Autodesk Inventor part; units mm, degrees
ref_plane "YZ Plane" through (0, 0, 0) normal (1, 0, 0) x (0, 1, 0)
ref_plane "XZ Plane" through (0, 0, 0) normal (0, 1, 0) x (-1, 0, 0)
ref_plane "XY Plane" through (0, 0, 0) normal (0, 0, 1) x (1, 0, 0)
sketch "Sketch1" plane through (0, 0, 0) normal (0, 0, 1) x (1, 0, 0)
  line L0 (-179.705, 0) -> (89.2175, 0)
  line L1 (0, -106.7147) -> (0, 106.7147)
  circle A0 centre (0, 0) radius 50.8 construction
  arc A1 (-12.7, 50.8248) -> (-12.7, -50.8248) centre (0, 0) ccw
  line L2 (0, -55.5625) -> (0, -68.2625)
  circle A2 centre (-101.6, 0) radius 14.2875
  line L3 (-101.6, -14.2875) -> (-101.6, 14.2875) construction
  line L4 (-115.6934, 37.1008) -> (-12.7, 76.2248)
  line L5 (-115.6934, -37.1008) -> (-12.7, -76.2248)
  arc A3 (-115.6934, 37.1008) -> (-115.6934, -37.1008) centre (-101.6, 0) ccw
  line L6 (-12.7, 50.8248) -> (-12.7, 76.2248)
  line L7 (-12.7, -76.2248) -> (-12.7, -50.8248)
  dimension "d0" = 101.6
  dimension "d1" = 1.5875
  dimension "d2" = 28.575
  dimension "d4" = 101.6
  dimension "d7" = 25.4
  dimension "d8" = 25.4
  dimension "d10" = 12.7
extrude "Extrusion1" add sketch "Sketch1" along normal mid plane 6.35 contours A3 L4 L6 A1 L0 A2 | L0 A2 A1 L7 L5 A3
sketch "Sketch2" plane through (0, 0, 3.175) normal (0, 0, 1) x (1, 0, 0)
  line L0 (-12.7, 76.2248) -> (-12.7, 50.8248)
  line L1 (-167.005, 0) -> (13.0175, 0)
  point P0 (-22.225, 60.3498)
  point P1 (-22.225, -60.3498)
  dimension "d13" = 9.525
  dimension "d14" = 15.875
hole "Hole1" at (-22.225, 60.3498, 3.175) at (-22.225, -60.3498, 3.175) direction (0, 0, -1) diameter 5.1054 end through all counterbore diameter 9.779 counterbore depth 1.5875
fillet "Fillet1" radius 12.7 1 edges at (-12.7, 76.2248, 0)
fillet "Fillet1" radius 12.7 1 edges at (-12.7, -76.2248, 0)
sketch "Sketch3" plane through (0, 0, 3.175) normal (0, 0, 1) x (1, 0, 0)
  arc A0 (-115.6934, 37.1008) -> (-115.6934, -37.1008) centre (-101.6, 0) ccw
  line L0 (-169.545, 0) -> (28.2575, 0)
  point P0 (-101.6, 34.925)
  point P1 (-101.6, -34.925)
  dimension "d24" = 34.925
hole "Hole2" at (-101.6, 34.925, 3.175) at (-101.6, -34.925, 3.175) direction (0, 0, -1) diameter 5.1054 end through all counterbore diameter 9.779 counterbore depth 1.5875
properties part number "plate2"
Check sheet for the modelled part. Datum: model origin and axes. Units: mm. A direction names the side the tool comes from. Round coordinates to 2 decimals unless told otherwise and drop trailing zeros. Loops run counter-clockwise (first coordinate to the right, second up) from the corner with the lowest first, then second, coordinate; pieces in that order, holes last. Notation, with made-up numbers: M -17,68.25 L -12,68.25 A29 ccw -12,89.25 Z; hole C 31.25,-40 d4. An arc over 180 degrees is marked long. One line per item, written item: value.
(1) Sectioned sample at C-C, the plane z = -2. Record the cut outline in (x, y) (1 decimal).
Computed values:
outline: M -115.7,-37.1 L -29.9,-69.7 A12.7 ccw -12.7,-57.8 L -12.7,-50.8 A52.4 cw -12.7,50.8 L -12.7,57.8 A12.7 ccw -29.9,69.7 L -115.7,37.1 A39.7 ccw Z; hole C -101.6,0 d28.6; hole C -101.6,-34.9 d5.1; hole C -101.6,34.9 d5.1; hole C -22.2,-60.3 d5.1; hole C -22.2,60.3 d5.1
(2) Sectioned sample at B-B, the plane x = -94. Record the cut outline in (y, z) (3 decimals), then the cut area to 3 significant figures.
Computed values:
outline: M -45.341,-3.175 L -12.098,-3.175 L -12.098,3.175 L -45.341,3.175 Z; M 12.098,-3.175 L 45.341,-3.175 L 45.341,3.175 L 12.098,3.175 Z
area: 422 mm^2
(3) Thickness scan on line 1 (Y direction, x = -101.6, z = -0.8); line 2 (Y direction, x = -101.6, z = 2.3); line 3 (Y direction, x = -110.5, z = 0.5). Record the ranges inside material, lowest first.
Computed values:
line 1: y = -42.45 to -37.48, -32.37 to -14.29, 14.29 to 32.37, 37.48 to 42.45
line 2: y = -42.45 to -39.81, -30.04 to -14.29, 14.29 to 30.04, 39.81 to 42.45
line 3: y = -39.07 to -11.18, 11.18 to 39.07
(4) Release check for a two-part mould opening along X. For faces 3 (the face through (-98.625, -31.045, 2.37)), 4 (the face through (-52.38, -0.97, -0.04)), 5 (the face through (-78, 1, -3.175)) record: +X half, -X half, draft (parallel to the pull), parting line (faces both ways), or undercut.
Computed values:
face 3: undercut
face 4: +X half
face 5: draft
(5) Depth check by flat-ended pin: pin 1 Ø2 at (x, z) = (-31, 1) entering from -Y; pin 2 Ø5 at (x, y) = (-20.5, -61.5) entering from +Z; pin 3 Ø3 at (x, y) = (-101.6, -34.925) entering from -Z; pin 4 Ø2 at (y, z) = (34, 2) entering from +X. Enter the tip coordinate at first touch or a pass-through.
Computed values:
pin 1: stops at y = -69.65
pin 2: stops at z = 1.59
pin 3: passes through
pin 4: stops at x = -38.98
(6) Sectioned sample at D-D, the plane x = -69.5. Record the cut outline in (y, z) (3 decimals), then the cut area to 3 significant figures.
Computed values:
outline: M -54.648,-3.175 L 54.648,-3.175 L 54.648,3.175 L -54.648,3.175 Z
area: 694 mm^2
(7) Access from +Z, -Z, +X, -X, +Y, -Y to the whole of each face (thin tool, end or side, straight path). Record for faces 1 (the face through (-12.7, -54, 0)), 2 (the face through (-99, 33, 1.588)).
Computed values:
face 1: +Z, -Z, +X, +Y, -Y
face 2: +Z
(8) Sectioned sample at A-A, the plane y = 0. Record the cut outline in (x, z) (1 decimal), then the cut area to 3 significant figures.
Computed values:
outline: M -141.3,-3.2 L -115.9,-3.2 L -115.9,3.2 L -141.3,3.2 Z; M -87.3,-3.2 L -52.4,-3.2 L -52.4,3.2 L -87.3,3.2 Z
area: 383 mm^2
